Geometry check sheet. Reference: the model listing, model coordinates, mm. Give positions to 0.01 mm unless a question says otherwise; leave off trailing zeros. Loops run counter-clockwise (first coordinate to the right, second up) from the corner with the lowest first, then second, coordinate; pieces in that order, holes last. Notation, with made-up numbers: (49.25, 64.25) -> (77.25, 64.25) arc R30 ccw to (77.25, 99.25) -> close; hole circle Ø7 at (72, -26.5). An arc over 180 degrees is marked (long way). Answer as a JSON object with one key per item and string values.
Autodesk Inventor part; units mm, degrees
ref_plane "YZ Plane" through (0, 0, 0) normal (1, 0, 0) x (0, 1, 0)
ref_plane "XZ Plane" through (0, 0, 0) normal (0, 1, 0) x (-1, 0, 0)
ref_plane "XY Plane" through (0, 0, 0) normal (0, 0, 1) x (1, 0, 0)
sketch "Sketch1" plane through (0, 0, 0) normal (0, 1, 0) x (-1, 0, 0)
  line L0 (0, 0) -> (152.4, 0) construction
  line L1 (152.4, 0) -> (152.4, -152.4) construction
  line L2 (152.4, -152.4) -> (0, -152.4) construction
  line L3 (0, -152.4) -> (0, 0) construction
  line L4 (44.6369, -152.4) -> (0, -107.7631) construction
  line L5 (0, -107.7631) -> (0, -44.6369) construction
  line L6 (0, -44.6369) -> (44.6369, 0) construction
  line L7 (44.6369, 0) -> (107.7631, 0) construction
  line L8 (107.7631, 0) -> (152.4, -44.6369) construction
  line L9 (152.4, -44.6369) -> (152.4, -107.7631) construction
  line L10 (152.4, -107.7631) -> (107.7631, -152.4) construction
  line L11 (107.7631, -152.4) -> (44.6369, -152.4) construction
  line L12 (102.5026, -12.7) -> (139.7, -49.8974) construction
  line L13 (139.7, -49.8974) -> (139.7, -102.5026) construction
  line L14 (139.7, -102.5026) -> (102.5026, -139.7) construction
  line L15 (102.5026, -139.7) -> (49.8974, -139.7) construction
  line L16 (49.8974, -139.7) -> (12.7, -102.5026) construction
  line L17 (12.7, -102.5026) -> (12.7, -49.8974) construction
  line L18 (12.7, -49.8974) -> (49.8974, -12.7) construction
  line L19 (49.8974, -12.7) -> (102.5026, -12.7) construction
  line L20 (152.4, -44.6369) -> (139.7, -49.8974)
  line L21 (139.7, -49.8974) -> (139.7, -102.5026)
  line L22 (152.4, -107.7631) -> (139.7, -102.5026)
  line L23 (152.4, -107.7631) -> (152.4, -44.6369)
  point P0 (76.2, -76.2)
  point P1 (76.2, -76.2)
  point P2 (76.2, -76.2)
  dimension "d0" = 152.4
  dimension "d1" = 152.4
  dimension "d2" = 12.7
  dimension "d3" = 63.1262
  dimension "d4" = 52.6051
extrude "Extrusion1" add sketch "Sketch1" along normal blind 127
sketch "Sketch2" plane through (-152.4, 0, -107.7631) normal (-1, 0, 0) x (0, 0, 1)
  line L0 (63.1261, 0) -> (63.1261, 127)
  line L1 (0, 127) -> (63.1261, 127)
  line L2 (0, 0) -> (0, 127)
  line L3 (0, 0) -> (63.1261, 0)
  line L4 (12.7, 114.3) -> (50.4261, 114.3)
  line L5 (50.4261, 114.3) -> (50.4261, 12.7)
  line L6 (50.4261, 12.7) -> (12.7, 12.7)
  line L7 (12.7, 12.7) -> (12.7, 114.3)
  point P0 (107.7631, 0)
  point P1 (12.7, 12.7)
  dimension "d7" = 12.7
  dimension "d8" = 12.7
  dimension "d9" = 12.7
  dimension "d10" = 12.7
  dimension "d11" = 12.7
  dimension "d12" = 12.7
  dimension "d13" = 12.7
  dimension "d14" = 12.7
extrude "Extrusion2" cut sketch "Sketch2" against normal up to surface (12.7 mm away) contours L4 L5 L6 L7
sketch "Sketch4" plane through (-152.4, 0, -107.7631) normal (-1, 0, 0) x (0, 0, 1)
  line L0 (0, 127) -> (63.1261, 127)
  line L1 (0, 0) -> (0, 127)
  line L2 (0, 0) -> (63.1261, 0)
  line L3 (63.1261, 0) -> (63.1261, 127)
  line L4 (10.16, 116.84) -> (52.9661, 116.84)
  line L5 (52.9661, 116.84) -> (52.9661, 10.16)
  line L6 (52.9661, 10.16) -> (10.16, 10.16)
  line L7 (10.16, 10.16) -> (10.16, 116.84)
  line L8 (50.4261, 114.3) -> (12.7, 114.3)
  line L9 (50.4261, 114.3) -> (50.4261, 12.7)
  line L10 (12.7, 114.3) -> (50.4261, 114.3)
  line L11 (50.4261, 114.3) -> (50.4261, 12.7)
  line L12 (50.4261, 12.7) -> (12.7, 12.7)
  line L13 (12.7, 12.7) -> (12.7, 114.3)
  point P0 (107.7631, 0)
  dimension "d17" = 10.16
  dimension "d18" = 10.16
  dimension "d19" = 10.16
  dimension "d20" = 10.16
extrude "Extrusion3" cut sketch "Sketch4" against normal blind 6.35 contours L4 L5 L6 L7
equation "\"d9\" = d8"
equation "\"d10\" = d8"
equation "\"d13\" = d9"
equation "\"d14\" = d9"
properties part number "SatelliteSideWallSensor"
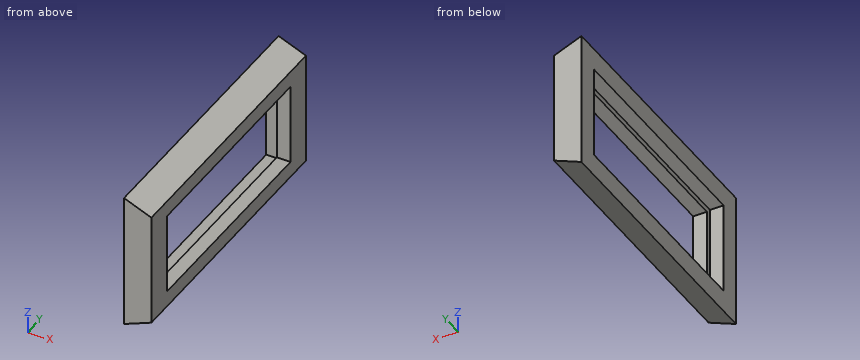
1) Section check A-A on y = 52. Record the cut outline in (x, z), plus the area to 3 significant figures.
Geometry check:
{"outline": "(-152.4, -107.76) -> (-139.7, -102.5) -> (-139.7, -95.06) -> (-146.05, -95.06) -> (-146.05, -97.6) -> (-152.4, -97.6) -> close; (-152.4, -54.8) -> (-146.05, -54.8) -> (-146.05, -57.34) -> (-139.7, -57.34) -> (-139.7, -49.9) -> (-152.4, -44.64) -> close", "area": "224 mm2"}
2) Section check B-B on z = -82. Record the cut outline in (x, y), plus the area to 3 significant figures.
Geometry check:
{"outline": "(-152.4, 0) -> (-139.7, 0) -> (-139.7, 12.7) -> (-146.05, 12.7) -> (-146.05, 10.16) -> (-152.4, 10.16) -> close; (-152.4, 116.84) -> (-146.05, 116.84) -> (-146.05, 114.3) -> (-139.7, 114.3) -> (-139.7, 127) -> (-152.4, 127) -> close", "area": "290 mm2"}
3) Section check D-D on y = 115.5. Record the cut outline in (x, z).
Geometry check:
{"outline": "(-152.4, -107.76) -> (-139.7, -102.5) -> (-139.7, -49.9) -> (-152.4, -44.64) -> (-152.4, -54.8) -> (-146.05, -54.8) -> (-146.05, -97.6) -> (-152.4, -97.6) -> close"}
4) Material ranges on line 1 along Y through (x, z) = (-146.25, -91); line 2 along Y through (x, z) = (-141.25, -91); line 3 along Z through (x, y) = (-142.75, 108.5), recorded low to high. Write a range as from..to.
Geometry check:
{"line 1": "y = 0..10.16, 116.84..127", "line 2": "y = 0..12.7, 114.3..127", "line 3": "z = -103.77..-95.06, -57.34..-48.63"}
5) Section check C-C on x = -141.25. Record the cut outline in (y, z), plus the area to 3 significant figures.
Geometry check:
{"outline": "(0, -103.14) -> (127, -103.14) -> (127, -49.26) -> (0, -49.26) -> close; hole (12.7, -95.06) -> (114.3, -95.06) -> (114.3, -57.34) -> (12.7, -57.34) -> close", "area": "3,010 mm2"}
6) Depth check by flat-ended pin: P1, Ø1.9, axis at x = -143, y = 45.5, coming from the -Z side; P2, Ø1.9, axis at x = -143.5, y = 55.5, coming from the +Z side; P3, Ø3, axis at x = -148, y = 112.5, coming from the -Z side. Enter the tip coordinate at first touch or a pass-through.
Geometry check:
{"P1": "stops at z = -104.26", "P2": "stops at z = -47.93", "P3": "stops at z = -106.56"}
